```python
from build123d import *

# Parameters (mm, degrees)
SKETCH4_R      = 2.031992692
SKETCH4_R_2    = 1.179287719
SKETCH4_R_3    = 1.905
SKETCH4_R_4    = 4.7244
EXTRUDE3_DEPTH = 4.7498


with BuildPart() as part:
    # Sketch4 → Extrude3 (new body)
    with BuildSketch(Plane.XY):
        with BuildLine():
            Line((-42.343481517, -2.990600597), (-42.343481517, 17.964399403))
            ThreePointArc((-42.343481517, 17.964399403), (-41.413545547, 20.209463433), (-39.168481517, 21.139399403))
            Line((-39.168481517, 21.139399403), (-15.038481517, 21.139399403))
            Line((-15.038481517, 21.139399403), (-15.038481517, 18.236569756))
            ThreePointArc((-15.038481517, 18.236569756), (-14.108545547, 15.991505726), (-11.863481517, 15.061569756))
            Line((-11.863481517, 15.061569756), (9.257081626, 15.061569756))
            ThreePointArc((9.257081626, 15.061569756), (11.502145656, 15.991505726), (12.432081626, 18.236569756))
            Line((12.432081626, 18.236569756), (12.432081626, 22.681569756))
            Line((12.432081626, 22.681569756), (52.437081626, 22.681569756))
            ThreePointArc((52.437081626, 22.681569756), (54.682145656, 21.751633786), (55.612081626, 19.506569756))
            Line((55.612081626, 19.506569756), (55.612081626, -9.945714332))
            ThreePointArc((55.612081626, -9.945714332), (56.542017596, -12.190778362), (58.787081626, -13.120714332))
            Line((58.787081626, -13.120714332), (61.618454053, -13.120714332))
            Line((61.618454053, -13.120714332), (61.618454053, -19.76149571))
            Line((61.618454053, -19.76149571), (12.432081626, -19.76149571))
            Line((12.432081626, -19.76149571), (12.432081626, -17.323430244))
            ThreePointArc((12.432081626, -17.323430244), (11.502145656, -15.078366214), (9.257081626, -14.148430244))
            Line((9.257081626, -14.148430244), (-18.530518374, -14.148430244))
            ThreePointArc((-18.530518374, -14.148430244), (-20.775582404, -15.078366214), (-21.705518374, -17.323430244))
            Line((-21.705518374, -17.323430244), (-21.705518374, -19.76149571))
            Line((-21.705518374, -19.76149571), (-40.618560355, -19.76149571))
            Line((-40.618560355, -19.76149571), (-40.618560355, -13.120714332))
            Line((-40.618560355, -13.120714332), (-35.040518374, -13.120714332))
            ThreePointArc((-35.040518374, -13.120714332), (-32.795454344, -12.190778362), (-31.865518374, -9.945714332))
            Line((-31.865518374, -9.945714332), (-31.865518374, -9.340600597))
            ThreePointArc((-31.865518374, -9.340600597), (-32.795454344, -7.095536567), (-35.040518374, -6.165600597))
            Line((-35.040518374, -6.165600597), (-39.168481517, -6.165600597))
            ThreePointArc((-39.168481517, -6.165600597), (-41.413545547, -5.235664628), (-42.343481517, -2.990600597))
        make_face()
        with Locations((-27.221195322, -14.622613425)):
            Circle(SKETCH4_R, mode=Mode.SUBTRACT)
        with Locations((-28.055981517, 6.851899403)):
            Circle(SKETCH4_R_2, mode=Mode.SUBTRACT)
        with Locations((52.287415303, -15.678066597)):
            Circle(SKETCH4_R_3, mode=Mode.SUBTRACT)
        with Locations((33.387081626, 0.456569756)):
            Circle(SKETCH4_R_4, mode=Mode.SUBTRACT)
        with Locations((13.846294556, -12.683763681)):
            Circle(SKETCH4_R_3, mode=Mode.SUBTRACT)
        with Locations((13.846294556, 13.596903192)):
            Circle(SKETCH4_R_3, mode=Mode.SUBTRACT)
        with Locations((-37.474326825, 16.270244711)):
            Circle(SKETCH4_R_3, mode=Mode.SUBTRACT)
        with Locations((-16.452694446, 13.596903192)):
            Circle(SKETCH4_R_3, mode=Mode.SUBTRACT)
        with Locations((50.814973838, 17.884461968)):
            Circle(SKETCH4_R_3, mode=Mode.SUBTRACT)
    extrude(amount=EXTRUDE3_DEPTH)


solid = part.part
```
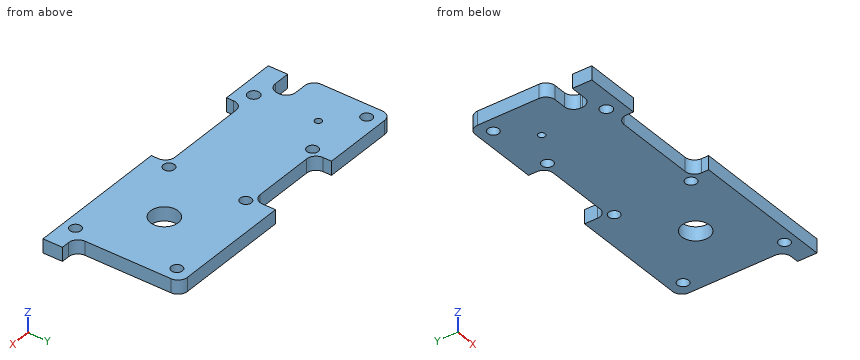
The model under review builds one solid part; all positions refer to its coordinate system, in mm. Coordinates: 2 decimals unless noted, no trailing zeros. Write each loop counter-clockwise with the first axis right and the second up, starting at its lowest first coordinate (ties: lowest second). Pieces come first, ordered by that corner, then holes. Notation, with made-up numbers: (48.25, 19.5) -> (67.25, 19.5) arc R24 cw to (67.25, 48.5) -> close; hole circle Ø7 at (5, 34). An arc over 180 degrees is marked (long way). One line per item, written item: value. Start each with the question number.
Q1. To check wall thickness, follow probe 1 along X at (y, z) = (-18, 2.5); probe 2 along X at (y, z) = (0.5, 2.3); probe 3 along X at (y, z) = (-13.5, 2.2). State the ranges of each line that lie inside material, in increasing order.
Q2. Clearance check with flat-ended pins moving along their axes: P1, Ø2.5, axis at y = 20.5, z = 2, coming from the +X side; P2, Ø8.5, axis at x = 33.39, y = 0.46, coming from the +Z side; P3, Ø2.5, axis at x = -22, z = 3.5, coming from the +Y side; P4, Ø2.5, axis at y = -18.5, z = 2.5, coming from the -X side. State where each tip first meets the part, or that it passes through.
Q3. Add section A-A, the plane x = -13.5. Give the boundary of the cut face in (y, z).
Q4. Add section B-B, the plane z = 1.8. Count the separate pieces of the cut face and the enclosed holes in it, then the cut area to 3 significant figures.
Response:
1. probe 1: -40.62 to -21.71, 12.43 to 61.62
1. probe 2: -42.34 to 28.66, 38.11 to 55.61
1. probe 3: -40.62 to -28.91, -25.53 to 12.13, 15.57 to 61.62
2. P1: x = 55.61
2. P2: through
2. P3: y = 21.14
2. P4: x = -40.62
3. outline: (-14.15, 0) -> (15.52, 0) -> (15.52, 4.75) -> (-14.15, 4.75) -> close
4. separate pieces: 1
4. enclosed holes: 9
4. area: 3,520 mm²
